Design review of the part built by this model. Coordinates are the model's own, in mm. Face numbers are marked on the shaded views. Coordinates: 2 decimals unless noted, no trailing zeros. Loops run counter-clockwise (first coordinate to the right, second up) from the corner with the lowest first, then second, coordinate; pieces in that order, holes last. Notation, with made-up numbers: M 17.25,84.25 L 65.25,84.25 A24 cw 65.25,107.25 Z; hole C -7,57.5 d3. An arc over 180 degrees is marked long. Answer as a JSON object with one key per item and string values. Group by question number.
1. Insertion check: pin 1 (3 mm diameter, centred on y = 4.5, z = -3.5, fed in from +X); pin 2 (5.5 mm diameter, centred on y = 0, z = 0, fed in from +X); pin 3 (3 mm diameter, centred on x = 5.5, y = 2, fed in from +Z). Each pin has a flat end and moves straight along its axis. Give the tip position at first contact, or say it passes through.
2. Consider section D-D (y = -5). State the section outline as (x, z) points.
3. Consider section C-C (x = 4.5). State the section outline as (y, z) points (3 decimals), then the cut area to 3 significant figures.
4. To check wall thickness, follow probe 1 along Z at (x, y) = (4.25, 0) (3 decimals); probe 2 along X at (y, z) = (0, -4.75); probe 3 along Z at (x, y) = (4.5, -2.25). State the ranges of each line that lie inside material, in increasing order.
5. Consider section A-A (z = 0). State the section outline as (x, y) points (3 decimals), then the cut area to 3 significant figures.
6. Draft analysis for pull direction Y (two halves, no side actions). For the marked faces 1, 2 and 3, state which applies: +Y half, -Y half, draft (parallel to the pull), parting line (faces both ways), or undercut.
Autodesk Inventor part; units mm, degrees
ref_plane "YZ Plane" through (0, 0, 0) normal (1, 0, 0) x (0, 1, 0)
ref_plane "XZ Plane" through (0, 0, 0) normal (0, 1, 0) x (-1, 0, 0)
ref_plane "XY Plane" through (0, 0, 0) normal (0, 0, 1) x (1, 0, 0)
sketch "Sketch_1" plane through (0, 0, 0) normal (0, 0, 1) x (1, 0, 0)
  line L0 (7, 0) -> (0, 0)
  line L1 (0, 3.3) -> (0.3, 3)
  line L2 (0.3, 3) -> (6.7, 3)
  line L3 (6.7, 3) -> (7, 3.3)
  line L4 (7, 3.3) -> (7, 3.7)
  line L5 (7, 3.7) -> (6, 4)
  line L6 (6, 4) -> (1, 4)
  line L7 (1, 4) -> (1, 6)
  line L8 (1, 6) -> (0, 6)
  line L9 (0, 6) -> (0, 3.3)
revolve "Revolution1" add sketch "Sketch_1" angle 360 about axis through (7, 0, 0) along (1, 0, 0)
sketch "스케치2" plane through (0, 0, 0) normal (-1, 0, 0) x (0, 0, 1)
  circle A0 centre (0, 0) radius 3.3
  circle A1 centre (0, 0) radius 6
  circle A2 centre (0, 0) radius 3.025
  dimension "d1" = 6.05
extrude "돌출1" cut sketch "스케치2" against normal up to surface (7 mm away) contours A2
move faces "이동1" translate (-2, 0, 0) faces at (0, 5.0099, -0.7419) (0.0917, 3.1979, -0.2582) (1, 5.2365, -0.7977) (0.6667, 5.9223, -0.9625)
properties part number "80F-0608"
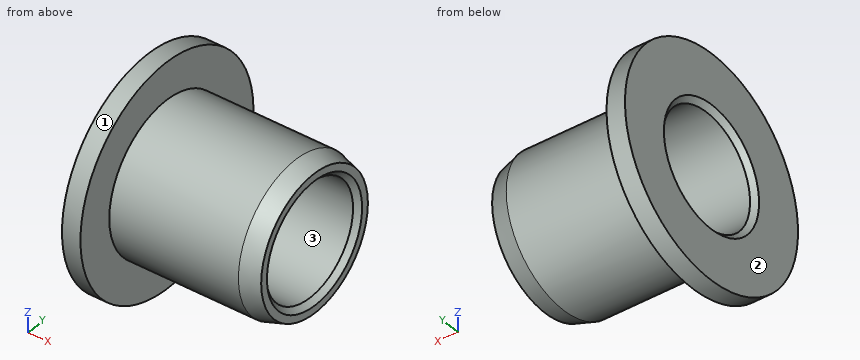
Findings below:
{
 "1": {"pin 1": "stops at x = -1", "pin 2": "passes through", "pin 3": "stops at z = 3.97"},
 "2": {"outline": "M -2,-3.32 L -1,-3.32 L -1,3.32 L -2,3.32 Z"},
 "3": {"outline": "C 0,0 d8; hole C 0,0 d6.05", "area": "21.5 mm^2"},
 "4": {"probe 1": "z = -4 to -3.025, 3.025 to 4", "probe 2": "x = -2 to -1", "probe 3": "z = -3.31 to -2.02, 2.02 to 3.31"},
 "5": {"outline": "M -2,-6 L -1,-6 L -1,-4 L 6,-4 L 7,-3.7 L 7,-3.3 L 6.725,-3.025 L -1.725,-3.025 L -2,-3.3 Z; M -2,3.3 L -1.725,3.025 L 6.725,3.025 L 7,3.3 L 7,3.7 L 6,4 L -1,4 L -1,6 L -2,6 Z", "area": "21.1 mm^2"},
 "6": {"face 1": "parting line", "face 2": "draft", "face 3": "undercut"}
}
